Work out the finished part from the listing and answer in its coordinate system (mm). A direction names the side the tool comes from. Round coordinates to 2 decimals unless told otherwise and drop trailing zeros. Write each loop counter-clockwise with the first axis right and the second up, starting at its lowest first coordinate (ties: lowest second). Pieces come first, ordered by that corner, then holes. Notation, with made-up numbers: (-7.75, 72) - (42.25, 72) arc R24 cw to (42.25, 110) - close; hole circle Ø7 at (84.5, -23.75). An arc over 180 degrees is marked (long way). Answer as a JSON object with one key per item and string values.
```python
from build123d import *

# Parameters (mm, degrees)
BOSS_EXTRUDE1_START = -342.9
SKETCH4_R           = 2.54
SKETCH4_R_2         = 14.2875
SKETCH4_R_3         = 9.525
BOSS_EXTRUDE1_DEPTH = 3.175
BOSS_EXTRUDE2_DEPTH = 3.175
BOSS_EXTRUDE3_START = -76.2
BOSS_EXTRUDE3_DEPTH = 3.175
SKETCH9_R           = 2.54
CUT_EXTRUDE2_DEPTH  = 523.969471233
LPATTERN1_COUNT     = 10
LPATTERN1_PITCH     = 50.8
SKETCH13_W          = 25.4
SKETCH13_H          = 139.7
CUT_EXTRUDE4_DEPTH  = 523.969471233


with BuildPart() as part:
    # Sketch4 → Boss-Extrude1 (new body)
    with BuildSketch(Plane(origin=(0, 0, 0), x_dir=(0, 0, -1), z_dir=(1, 0, 0)).offset(BOSS_EXTRUDE1_START)):
        with BuildLine():
            Line((363.380981673, 114.3), (0, 114.3))
            Line((0, 114.3), (0, 90.4875))
            ThreePointArc((0, 90.4875), (14.2875, 76.2), (0, 61.9125))
            Line((0, 61.9125), (0, 38.1))
            Line((0, 38.1), (363.380981673, 38.1))
            Line((363.380981673, 38.1), (363.380981673, 114.3))
        make_face()
        with Locations((53.34, 50.8)):
            Circle(SKETCH4_R, mode=Mode.SUBTRACT)
        with Locations((177.987401789, 57.15)):
            Circle(SKETCH4_R_2, mode=Mode.SUBTRACT)
        with Locations((53.34, 76.2)):
            Circle(SKETCH4_R_3, mode=Mode.SUBTRACT)
        with Locations((337.980981673, 60.325)):
            Circle(SKETCH4_R_2, mode=Mode.SUBTRACT)
        with Locations((53.34, 101.6)):
            Circle(SKETCH4_R, mode=Mode.SUBTRACT)
    extrude(amount=-BOSS_EXTRUDE1_DEPTH)

    # Sketch7 → Boss-Extrude2 (add)
    with BuildSketch(Plane(origin=(0, 114.3, 0), x_dir=(1, 0, 0), z_dir=(0, 1, 0))):
        Polygon((-344.4875, 0), (-368.3, 0), (-368.3, 363.380981673), (-342.9, 363.380981673), align=None)
    extrude(amount=-BOSS_EXTRUDE2_DEPTH)

    # Sketch7<2> → Boss-Extrude3 (add)
    with BuildSketch(Plane(origin=(0, 114.3, 0), x_dir=(1, 0, 0), z_dir=(0, 1, 0)).offset(BOSS_EXTRUDE3_START)):
        Polygon((-344.4875, 0), (-368.3, 0), (-368.3, 363.380981673), (-342.9, 363.380981673), align=None)
    extrude(amount=BOSS_EXTRUDE3_DEPTH)

    # Sketch9 → Cut-Extrude2 (cut, through all)
    with BuildSketch(Plane(origin=(0, 114.3, 0), x_dir=(1, 0, 0), z_dir=(0, 1, 0))):
        with Locations(Location((-355.6, 355.6, 0), (0, 0, 270))):
            Circle(SKETCH9_R)
    cut_extrude2 = extrude(amount=-CUT_EXTRUDE2_DEPTH, mode=Mode.SUBTRACT)

    # LPattern1: Cut-Extrude2 ×10
    with Locations(*[(0, 0, i * LPATTERN1_PITCH) for i in range(1, LPATTERN1_COUNT)]):
        add(cut_extrude2, mode=Mode.SUBTRACT)

    # Mirror1: part across face


with BuildPart() as part_1:
    add(part.part)
    add(part.part.mirror(Plane(origin=(-345.639664948, 104.734085052, 0), x_dir=(1, 0, 0), z_dir=(0, 0, 1))))

    # Sketch13 → Cut-Extrude4 (cut, through all)
    with BuildSketch(Plane(origin=(0, 114.3, 0), x_dir=(1, 0, 0), z_dir=(0, 1, 0))):
        with Locations((-355.6, 293.530981673)):
            Rectangle(SKETCH13_W, SKETCH13_H)
        with Locations((-355.6, -293.530981673)):
            Rectangle(SKETCH13_W, SKETCH13_H)
    extrude(amount=-CUT_EXTRUDE4_DEPTH, mode=Mode.SUBTRACT)


solid = part_1.part
```
Item 1: For faces 1 (the flat face through (-357, 111.125, 3)), 2 (the flat face through (-355, 38.1, -3)), determine the directions among +Z, -Z, +X, -X, +Y, -Y from which every point of the face is accessible in a straight line to the end or side of a thin tool.
Results found:
{"face 1": "+Z, -Z, -X", "face 2": "+Z, -Z, +X, -X, -Y"}
Item 2: Each of these flat-tipped pins is pushed along its axis until it touches: P1, Ø4, axis at x = -355.6, z = -50.8, coming from the -Y side; P2, Ø6, axis at y = 50.8, z = -53.34, coming from the +X side; P3, Ø1, axis at y = 91, z = 40.5, coming from the -X side (3 decimals). Where does it stop, or does it pass through?
Results found:
{"P1": "through", "P2": "x = -342.9", "P3": "x = -346.075"}
Item 3: A cutting plane is placed at B-B (y = 57.15). Write down the section's boundary in (x, z) (3 decimals).
Results found:
{"outline": "(-346.075, -223.681) - (-342.9, -223.681) - (-342.9, -192.275) - (-346.075, -192.275) - close; (-346.075, -163.7) - (-342.9, -163.7) - (-342.9, 163.7) - (-346.075, 163.7) - close; (-346.075, 192.275) - (-342.9, 192.275) - (-342.9, 223.681) - (-346.075, 223.681) - close"}
Item 4: A cutting plane is placed at D-D (z = -183). Write down the section's boundary in (x, y) (3 decimals), and give its area (3 significant figures).
Results found:
{"outline": "(-368.3, 38.1) - (-342.9, 38.1) - (-342.9, 43.771) - (-346.075, 43.771) - (-346.075, 41.275) - (-368.3, 41.275) - close; (-368.3, 111.125) - (-346.075, 111.125) - (-346.075, 70.529) - (-342.9, 70.529) - (-342.9, 114.3) - (-368.3, 114.3) - close", "area": "298 mm²"}
Item 5: Determine the mould class of faces 3 (the flat face through (-345, 76, 223.681)), 4 (the flat face through (-346.075, 61, -3)), 5 (the cylindrical face through (-344.465, 57.778, 163.714)), 6 (the cylindrical face through (-344.47, 72.55, -62.14)) for opening direction Z: pulls with the +Z half, pulls with the -Z half, needs draft (parallel to the pull), parting line crosses it, or undercut.
Results found:
{"face 3": "pulls with the +Z half", "face 4": "needs draft", "face 5": "undercut", "face 6": "undercut"}
Item 6: A cutting plane is placed at C-C (z = -118). Write down the section's boundary in (x, y) (3 decimals).
Results found:
{"outline": "(-368.3, 38.1) - (-342.9, 38.1) - (-342.9, 114.3) - (-368.3, 114.3) - (-368.3, 111.125) - (-346.075, 111.125) - (-346.075, 41.275) - (-368.3, 41.275) - close"}
Item 7: Consider line 1 along Y through (x, z) = (-344, -53.34) (3 decimals); line 2 along Y through (x, z) = (-358.25, 38) (3 decimals); line 3 along X through (y, z) = (39, 101). Determine where each line is inside the solid, lowest interval first.
Results found:
{"line 1": "38.1 to 48.26, 53.34 to 66.675, 85.725 to 99.06, 104.14 to 114.3", "line 2": "38.1 to 41.275, 111.125 to 114.3", "line 3": "-368.3 to -358.07, -353.13 to -342.9"}
Item 8: A cutting plane is placed at A-A (y = 76.2). Write down the section's boundary in (x, z) (1 decimal).
Results found:
{"outline": "(-346.1, -223.7) - (-342.9, -223.7) - (-342.9, -62.9) - (-346.1, -62.9) - close; (-346.1, -43.8) - (-342.9, -43.8) - (-342.9, -14.3) - (-346.1, -14.3) - close; (-346.1, 14.3) - (-342.9, 14.3) - (-342.9, 43.8) - (-346.1, 43.8) - close; (-346.1, 62.9) - (-342.9, 62.9) - (-342.9, 223.7) - (-346.1, 223.7) - close"}
